CAD build for the part. Positions are in the model's coordinates, mm. A direction names the side the tool comes from. Give positions to 0.01 mm unless a question says otherwise; leave off trailing zeros. Order: outer loops, then holes, each group sorted by start corner. A loop starts at its lowest first (then second) coordinate and runs counter-clockwise, first axis right, second up. Notation, with made-up numbers: M -5,41.5 L 10,41.5 A12 ccw 10,49.5 Z; hole C -36.75,59 d5. An arc over 180 degrees is marked long. Put each result on its own line as item: value. Start each with the question number.
1) Drill centre lines: line 1 (Y direction, x = 4, z = 26); line 2 (X direction, y = 29, z = 46); line 3 (Y direction, x = 4, z = 32). Where is each one in solid material? Low to high. Write a range as [from, to].
2) Cut at A-A (x = 4). Write the cut outline in (y, z).
3) Two-plate mould, pull along X, no slides. Class faces 1 (the face through (29, 45, 60)), 2 (the face through (-3.791, 57.434, 29.58)), 3 (the face through (-9.843, 2.885, 29.58)): released by +X, released by -X, zero draft, split by the parting line, or undercut.
4) Cut at D-D (z = 50.5). Write the cut outline in (x, y).
5) Cut at C-C (y = 10). Write the cut outline in (x, z), and give its area (3 significant figures).
6) Pin check, flat tips, straight feed: pin 1 (1 mm diameter, centred on y = 38.5, z = 32.5, fed in from -X); pin 2 (2.5 mm diameter, centred on y = 28, z = 33, fed in from +X); pin 3 (6.5 mm diameter, centred on y = 38.5, z = 35.5, fed in from -X); pin 4 (5 mm diameter, centred on y = 30, z = 30.5, fed in from -X). Stop position of each tip, or through.
7) Tool access for faces 4 (the face through (0, 29, 34)), 5 (the face through (4, 45, 31)), 6 (the face through (7, 30, 38)): list every direction of +Z, -Z, +X, -X, +Y, -Y with a clear straight run to the whole face (end or side of a thin tool).
```python
from build123d import *

# Parameters (mm, degrees)
ESQUISSE1_W             = 8
ESQUISSE1_H             = 59
BOSS_EXTRU_1_DEPTH      = 60
ESQUISSE3_R             = 30
ESQUISSE3_R_2           = 29
BOSS_EXTRU_2_DEPTH      = 60
ESQUISSE4_R             = 29
ENL_V_MAT_EXTRU_3_DEPTH = 30
ENL_V_MAT_EXTRU_5_DEPTH = 1.5
ESQUISSE6_R             = 29
ENL_V_MAT_EXTRU_6_DEPTH = 22
ESQUISSE7_R             = 2
ENL_V_MAT_EXTRU_7_DEPTH = 6.5


with BuildPart() as part:
    # Esquisse1 → Boss.-Extru.1 (new body)
    with BuildSketch(Plane.XY):
        with Locations((4, 29.5)):
            Rectangle(ESQUISSE1_W, ESQUISSE1_H)
    extrude(amount=BOSS_EXTRU_1_DEPTH)

    # Esquisse3 → Boss.-Extru.2 (add)
    with BuildSketch(Plane(origin=(0, 0, 0), x_dir=(-1, 0, 0), z_dir=(0, 0, -1))):
        with Locations((-4, 29.5)):
            Circle(ESQUISSE3_R)
        with Locations((-4, 29.5)):
            Circle(ESQUISSE3_R_2, mode=Mode.SUBTRACT)
    extrude(amount=-BOSS_EXTRU_2_DEPTH)

    # Esquisse4 → Enlèv. mat.-Extru.3 (cut)
    with BuildSketch(Plane(origin=(0, 0, 0), x_dir=(-1, 0, 0), z_dir=(0, 0, -1))):
        with Locations((-4, 29.5)):
            Circle(ESQUISSE4_R)
    extrude(amount=-ENL_V_MAT_EXTRU_3_DEPTH, mode=Mode.SUBTRACT)

    # Esquisse5 → Enlèv. mat.-Extru.5 (cut)
    with BuildSketch(Plane(origin=(0, 0, 30), x_dir=(-1, 0, 0), z_dir=(0, 0, -1))):
        with BuildLine():
            Line((-6, 43), (-6.967257844, 29.9420191))
            ThreePointArc((-6.967257844, 29.9420191), (-7, 29.5), (-6.967257844, 29.0579809))
            Line((-6.967257844, 29.0579809), (-6, 16))
            ThreePointArc((-6, 16), (-4, 14), (-2, 16))
            Line((-2, 16), (-1.032742156, 29.0579809))
            ThreePointArc((-1.032742156, 29.0579809), (-1, 29.5), (-1.032742156, 29.9420191))
            Line((-1.032742156, 29.9420191), (-2, 43))
            ThreePointArc((-2, 43), (-4, 45), (-6, 43))
        make_face()
    extrude(amount=-ENL_V_MAT_EXTRU_5_DEPTH, mode=Mode.SUBTRACT)

    # Esquisse6 → Enlèv. mat.-Extru.6 (cut)
    with BuildSketch(Plane.XY.offset(60)):
        with Locations((4, 29.5)):
            Circle(ESQUISSE6_R)
    extrude(amount=-ENL_V_MAT_EXTRU_6_DEPTH, mode=Mode.SUBTRACT)

    # Esquisse7 → Enlèv. mat.-Extru.7 (cut)
    with BuildSketch(Plane(origin=(0, 0, 31.5), x_dir=(-1, 0, 0), z_dir=(0, 0, -1))):
        with Locations((-4, 29.5)):
            Circle(ESQUISSE7_R)
    extrude(amount=-ENL_V_MAT_EXTRU_7_DEPTH, mode=Mode.SUBTRACT)


solid = part.part
```
Solution:
1. line 1: [-0.5, 0.5], [58.5, 59.5]
1. line 2: [-26, -25], [33, 34]
1. line 3: [-0.5, 27.5], [31.5, 59.5]
2. outline: M -0.5,0 L 0.5,0 L 0.5,30 L 14,30 L 14,31.5 L 27.5,31.5 L 27.5,38 L 0.5,38 L 0.5,60 L -0.5,60 Z; M 31.5,31.5 L 45,31.5 L 45,30 L 58.5,30 L 58.5,0 L 59.5,0 L 59.5,60 L 58.5,60 L 58.5,38 L 31.5,38 Z
3. face 1: zero draft
3. face 2: undercut
3. face 3: split by the parting line
4. outline: C 4,29.5 d60; hole C 4,29.5 d58
5. outline: M -18.8,0 L -17.47,0 L -17.47,60 L -18.8,60 Z; M 0,30 L 8,30 L 8,38 L 0,38 Z; M 25.47,0 L 26.8,0 L 26.8,60 L 25.47,60 Z
5. area: 224 mm²
6. pin 1: x = -24.77
6. pin 2: x = 34
6. pin 3: x = -25.44
6. pin 4: x = -26
7. face 4: +Z, -Z
7. face 5: -Z
7. face 6: +Z
